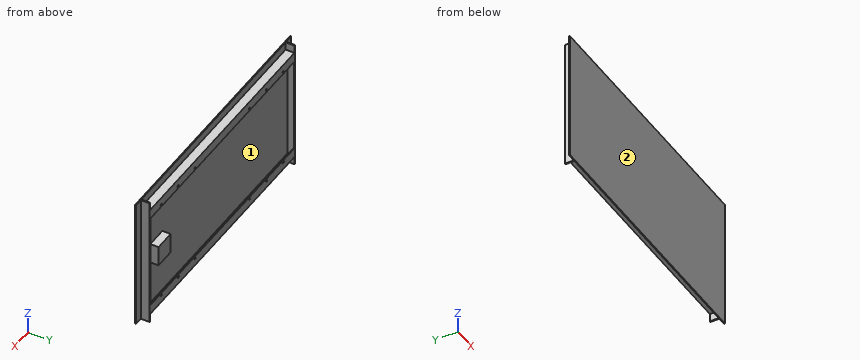
from build123d import *

# Parameters (mm, degrees)
SKETCH1_W            = 754.38
SKETCH1_H            = 351.155
BOSS_EXTRUDE1_DEPTH  = 9.525
SKETCH5_W            = 355.6
SKETCH5_H            = 30.1625
BOSS_EXTRUDE4_DEPTH  = 2.2225
SKETCH6_W            = 754.38
SKETCH6_H            = 30.1625
BOSS_EXTRUDE5_DEPTH  = 2.2225
SKETCH8_W            = 754.38
SKETCH8_H            = 30.1625
BOSS_EXTRUDE6_DEPTH  = 2.2225
SKETCH14_W           = 355.6
SKETCH14_H           = 30.1625
BOSS_EXTRUDE7_DEPTH  = 2.2225
SKETCH16_W           = 754.38
SKETCH16_H           = 2.2225
BOSS_EXTRUDE8_DEPTH  = 25.0825
SKETCH17_W           = 754.38
SKETCH17_H           = 2.2225
BOSS_EXTRUDE9_DEPTH  = 25.0825
CUT_EXTRUDE1_DEPTH   = 2.2225
SKETCH21_R           = 3.175
CUT_EXTRUDE3_DEPTH   = 2.2225
SKETCH22_W           = 758.825
SKETCH22_H           = 30.1625
BOSS_EXTRUDE10_DEPTH = 3.175
SKETCH23_W           = 758.825
SKETCH23_H           = 3.175
BOSS_EXTRUDE11_DEPTH = 25.4
SKETCH24_W           = 758.825
SKETCH24_H           = 30.1625
BOSS_EXTRUDE12_DEPTH = 3.175
SKETCH25_W           = 758.825
SKETCH25_H           = 3.175
BOSS_EXTRUDE13_DEPTH = 25.4
SKETCH26_W           = 412.75
SKETCH26_H           = 30.1625
BOSS_EXTRUDE14_DEPTH = 3.175
SKETCH27_W           = 412.75
SKETCH27_H           = 3.175
BOSS_EXTRUDE15_DEPTH = 25.4
SKETCH28_W           = 412.75
SKETCH28_H           = 30.1625
BOSS_EXTRUDE16_DEPTH = 3.175
SKETCH29_W           = 412.75
SKETCH29_H           = 3.175
BOSS_EXTRUDE17_DEPTH = 25.4
SKETCH30_W           = 63.5
SKETCH30_H           = 63.5
BOSS_EXTRUDE18_DEPTH = 25.4


with BuildPart() as part:
    # Sketch1 → Boss-Extrude1 (new body)
    with BuildSketch(Plane(origin=(0, 0, 0), x_dir=(1, 0, 0), z_dir=(0, 1, 0))):
        Rectangle(SKETCH1_W, SKETCH1_H)
    extrude(amount=BOSS_EXTRUDE1_DEPTH)

    # Sketch5 → Boss-Extrude4 (add)
    with BuildSketch(Plane.ZY.offset(377.19)):
        with Locations((0, 15.08125)):
            Rectangle(SKETCH5_W, SKETCH5_H)
    extrude(amount=BOSS_EXTRUDE4_DEPTH)

    # Sketch6 → Boss-Extrude5 (add)
    with BuildSketch(Plane.XY.offset(175.5775)):
        with Locations((0, 15.08125)):
            Rectangle(SKETCH6_W, SKETCH6_H)
    extrude(amount=BOSS_EXTRUDE5_DEPTH)

    # Sketch8 → Boss-Extrude6 (add)
    with BuildSketch(Plane(origin=(0, 0, -175.5775), x_dir=(-1, 0, 0), z_dir=(0, 0, -1))):
        with Locations((0, 15.08125)):
            Rectangle(SKETCH8_W, SKETCH8_H)
    extrude(amount=BOSS_EXTRUDE6_DEPTH)

    # Sketch14 → Boss-Extrude7 (add)
    with BuildSketch(Plane(origin=(377.19, 0, 0), x_dir=(0, 0, -1), z_dir=(1, 0, 0))):
        with Locations((0, 15.08125)):
            Rectangle(SKETCH14_W, SKETCH14_H)
    extrude(amount=BOSS_EXTRUDE7_DEPTH)

    # Sketch16 → Boss-Extrude8 (add)
    with BuildSketch(Plane.XY.offset(-175.5775)):
        with Locations((0, 29.05125)):
            Rectangle(SKETCH16_W, SKETCH16_H)
    extrude(amount=BOSS_EXTRUDE8_DEPTH)

    # Sketch17 → Boss-Extrude9 (add)
    with BuildSketch(Plane(origin=(0, 0, 175.5775), x_dir=(-1, 0, 0), z_dir=(0, 0, -1))):
        with Locations((0, 29.05125)):
            Rectangle(SKETCH17_W, SKETCH17_H)
    extrude(amount=BOSS_EXTRUDE9_DEPTH)

    # Sketch19 → Cut-Extrude1 (cut)
    with BuildSketch(Plane(origin=(0, 30.1625, 0), x_dir=(1, 0, 0), z_dir=(0, 1, 0))):
        with BuildLine():
            Line((-228.727, 157.1625), (-228.727, 158.4325))
            ThreePointArc((-228.727, 158.4325), (-231.902, 161.6075), (-235.077, 158.4325))
            Line((-235.077, 158.4325), (-235.077, 157.1625))
            ThreePointArc((-235.077, 157.1625), (-231.902, 153.9875), (-228.727, 157.1625))
        make_face()
        with BuildLine():
            Line((-235.077, -158.4325), (-235.077, -157.1625))
            ThreePointArc((-235.077, -157.1625), (-231.902, -153.9875), (-228.727, -157.1625))
            Line((-228.727, -157.1625), (-228.727, -158.4325))
            ThreePointArc((-228.727, -158.4325), (-231.902, -161.6075), (-235.077, -158.4325))
        make_face()
        with BuildLine():
            Line((228.727, -157.1625), (228.727, -158.4325))
            ThreePointArc((228.727, -158.4325), (231.902, -161.6075), (235.077, -158.4325))
            Line((235.077, -158.4325), (235.077, -157.1625))
            ThreePointArc((235.077, -157.1625), (231.902, -153.9875), (228.727, -157.1625))
        make_face()
        with BuildLine():
            Line((228.727, 157.1625), (228.727, 158.4325))
            ThreePointArc((228.727, 158.4325), (231.902, 161.6075), (235.077, 158.4325))
            Line((235.077, 158.4325), (235.077, 157.1625))
            ThreePointArc((235.077, 157.1625), (231.902, 153.9875), (228.727, 157.1625))
        make_face()
    extrude(amount=-CUT_EXTRUDE1_DEPTH, mode=Mode.SUBTRACT)

    # Sketch21 → Cut-Extrude3 (cut)
    with BuildSketch(Plane(origin=(0, 30.1625, 0), x_dir=(1, 0, 0), z_dir=(0, 1, 0))):
        with Locations(Location((-143.002, -157.1625, 0), (0, 0, 270))):
            Circle(SKETCH21_R)
        with Locations(Location((-143.002, 157.1625, 0), (0, 0, 270))):
            Circle(SKETCH21_R)
        with Locations(Location((-320.802, -157.1625, 0), (0, 0, 270))):
            Circle(SKETCH21_R)
        with Locations(Location((-320.802, 157.1625, 0), (0, 0, 270))):
            Circle(SKETCH21_R)
        with Locations(Location((143.002, 157.1625, 0), (0, 0, 270))):
            Circle(SKETCH21_R)
        with Locations(Location((320.802, 157.1625, 0), (0, 0, 270))):
            Circle(SKETCH21_R)
        with Locations(Location((143.002, -157.1625, 0), (0, 0, 270))):
            Circle(SKETCH21_R)
        with Locations(Location((320.802, -157.1625, 0), (0, 0, 270))):
            Circle(SKETCH21_R)
    extrude(amount=-CUT_EXTRUDE3_DEPTH, mode=Mode.SUBTRACT)

    # Sketch22 → Boss-Extrude10 (add)
    with BuildSketch(Plane.XY.offset(177.8)):
        with Locations((0, 15.08125)):
            Rectangle(SKETCH22_W, SKETCH22_H)
    extrude(amount=BOSS_EXTRUDE10_DEPTH)

    # Sketch23 → Boss-Extrude11 (add)
    with BuildSketch(Plane.XY.offset(180.975)):
        with Locations((0, 1.5875)):
            Rectangle(SKETCH23_W, SKETCH23_H)
    extrude(amount=BOSS_EXTRUDE11_DEPTH)

    # Sketch24 → Boss-Extrude12 (add)
    with BuildSketch(Plane(origin=(0, 0, -177.8), x_dir=(-1, 0, 0), z_dir=(0, 0, -1))):
        with Locations((0, 15.08125)):
            Rectangle(SKETCH24_W, SKETCH24_H)
    extrude(amount=BOSS_EXTRUDE12_DEPTH)

    # Sketch25 → Boss-Extrude13 (add)
    with BuildSketch(Plane(origin=(0, 0, -180.975), x_dir=(-1, 0, 0), z_dir=(0, 0, -1))):
        with Locations((0, 1.5875)):
            Rectangle(SKETCH25_W, SKETCH25_H)
    extrude(amount=BOSS_EXTRUDE13_DEPTH)

    # Sketch26 → Boss-Extrude14 (add)
    with BuildSketch(Plane.ZY.offset(379.4125)):
        with Locations((0, 15.08125)):
            Rectangle(SKETCH26_W, SKETCH26_H)
    extrude(amount=BOSS_EXTRUDE14_DEPTH)

    # Sketch27 → Boss-Extrude15 (add)
    with BuildSketch(Plane.ZY.offset(382.5875)):
        with Locations((0, 1.5875)):
            Rectangle(SKETCH27_W, SKETCH27_H)
    extrude(amount=BOSS_EXTRUDE15_DEPTH)

    # Sketch28 → Boss-Extrude16 (add)
    with BuildSketch(Plane(origin=(379.4125, 0, 0), x_dir=(0, 0, -1), z_dir=(1, 0, 0))):
        with Locations((0, 15.08125)):
            Rectangle(SKETCH28_W, SKETCH28_H)
    extrude(amount=BOSS_EXTRUDE16_DEPTH)

    # Sketch29 → Boss-Extrude17 (add)
    with BuildSketch(Plane(origin=(382.5875, 0, 0), x_dir=(0, 0, -1), z_dir=(1, 0, 0))):
        with Locations((0, 1.5875)):
            Rectangle(SKETCH29_W, SKETCH29_H)
    extrude(amount=BOSS_EXTRUDE17_DEPTH)

    # Sketch30 → Boss-Extrude18 (add)
    with BuildSketch(Plane(origin=(0, 9.525, 0), x_dir=(1, 0, 0), z_dir=(0, 1, 0))):
        with Locations((311.785, 3.861461092)):
            Rectangle(SKETCH30_W, SKETCH30_H)
    extrude(amount=BOSS_EXTRUDE18_DEPTH)


solid = part.part
The model under review builds one solid part; all positions refer to its coordinate system, in mm. Face numbers are marked on the shaded views. Give positions to 0.01 mm unless a question says otherwise; leave off trailing zeros. Loops run counter-clockwise (first coordinate to the right, second up) from the corner with the lowest first, then second, coordinate; pieces in that order, holes last. Notation, with made-up numbers: (82.5, 88.5) -> (88.5, 88.5) arc R18 ccw to (88.5, 104.5) -> close; hole circle Ø3 at (73, 2.25). An arc over 180 degrees is marked (long way). Answer as a JSON object with one key per item and string values. Group by question number.
Q1. Wall thickness on line 1 along Z through (x, y) = (314.5, 16) (1 decimal); line 2 along X through (y, z) = (27.5, -35.5) (1 decimal); line 3 along Z through (x, y) = (63.5, 26) (1 decimal): over which ranges is each line inside the solid? List them lowest first.
Q2. Take a section at B-B (x = -339). Write out the cut boundary in (y, z) (1 decimal).
Q3. Draft analysis for pull direction X (two halves, no side actions). For the marked faces 1 and 2, state which applies: pulls with the +X half, pulls with the -X half, needs draft (parallel to the pull), parting line crosses it, or undercut.
Q4. Take a section at C-C (z = -84.5). Write out the cut boundary in (x, y) (1 decimal).
Q5. Take a section at A-A (y = 21). Write out the cut boundary in (x, z) (1 decimal), plus the area to 3 significant figures.
Q6. Insertion check: pin 1 (10.5 mm diameter, centred on y = 24, z = -71, fed in from -X); pin 2 (7.5 mm diameter, centred on x = -320.8, z = 157.16, fed in from +Y); pin 3 (9 mm diameter, centred on x = -140, y = 16, fed in from -Z) (3 decimals). Each pin has a flat end and moves straight along its axis. Give the tip position at first contact, or say it passes through.
Q7. Take a section at D-D (z = -12). Write out the cut boundary in (x, y) (1 decimal).
Answer below:
{
 "1": {"line 1": "z = -181 to -175.6, -35.6 to 27.9, 175.6 to 181", "line 2": "x = -382.6 to -377.2, 280 to 343.5, 377.2 to 382.6", "line 3": "z = -181 to -175.6, 175.6 to 181"},
 "2": {"outline": "(0, -206.4) -> (3.2, -206.4) -> (3.2, -181) -> (30.2, -181) -> (30.2, -150.5) -> (27.9, -150.5) -> (27.9, -175.6) -> (9.5, -175.6) -> (9.5, 175.6) -> (27.9, 175.6) -> (27.9, 150.5) -> (30.2, 150.5) -> (30.2, 181) -> (3.2, 181) -> (3.2, 206.4) -> (0, 206.4) -> close"},
 "3": {"face 1": "undercut", "face 2": "needs draft"},
 "4": {"outline": "(-408, 0) -> (408, 0) -> (408, 3.2) -> (382.6, 3.2) -> (382.6, 30.2) -> (377.2, 30.2) -> (377.2, 9.5) -> (-377.2, 9.5) -> (-377.2, 30.2) -> (-382.6, 30.2) -> (-382.6, 3.2) -> (-408, 3.2) -> close"},
 "5": {"outline": "(-382.6, -206.4) -> (-379.4, -206.4) -> (-379.4, -181) -> (379.4, -181) -> (379.4, -206.4) -> (382.6, -206.4) -> (382.6, 206.4) -> (379.4, 206.4) -> (379.4, 181) -> (-379.4, 181) -> (-379.4, 206.4) -> (-382.6, 206.4) -> close; (280, -35.6) -> (343.5, -35.6) -> (343.5, 27.9) -> (280, 27.9) -> close; hole (-377.2, -175.6) -> (377.2, -175.6) -> (377.2, 175.6) -> (-377.2, 175.6) -> close", "area": "16,400 mm2"},
 "6": {"pin 1": "stops at x = -382.59", "pin 2": "stops at y = 30.16", "pin 3": "stops at z = -180.975"},
 "7": {"outline": "(-408, 0) -> (408, 0) -> (408, 3.2) -> (382.6, 3.2) -> (382.6, 30.2) -> (377.2, 30.2) -> (377.2, 9.5) -> (343.5, 9.5) -> (343.5, 34.9) -> (280, 34.9) -> (280, 9.5) -> (-377.2, 9.5) -> (-377.2, 30.2) -> (-382.6, 30.2) -> (-382.6, 3.2) -> (-408, 3.2) -> close"}
}
